Geometry check sheet. Reference: the model listing, model coordinates, mm. Coordinates: 2 decimals unless noted, no trailing zeros. Order: outer loops, then holes, each group sorted by start corner. A loop starts at its lowest first (then second) coordinate and runs counter-clockwise, first axis right, second up. Notation, with made-up numbers: M 42.25,53 L 91.25,53 A18 ccw 91.25,83 Z; hole C -27,-10 d9. An arc over 180 degrees is marked long. One line per item, written item: value. Start each with the question number.
1) Sectioned sample at A-A, the plane x = 0. Enter the section's corners in (y, z) (3 decimals), then the cut area to 3 significant figures.
2) Sectioned sample at B-B, the plane z = 0. Enter the section's corners in (x, y) (3 decimals), then the cut area to 3 significant figures.
3) Go/stop test with flat-tipped pins: P1, Ø2, axis at y = 1, z = -3.5, coming from the -X side; P2, Ø1, axis at y = -1, z = -2.5, coming from the +X side; P3, Ø1, axis at x = 1, y = 0.5, coming from the +Z side. Record where each tip stops, or that it passes through.
4) Thickness scan on L1, parallel to Z at x = 0, y = -0.2; L2, parallel to X at y = -1.1, z = 1.5. Record the ranges inside material, lowest first. Write a range as from..to.
5) Sectioned sample at C-C, the plane y = -0.15. Enter the section's corners in (x, z).
6) Draft check along X on faces 1 (the cylindrical face through (0, 0, 2)), 2 (the cylindrical face through (-1.08, 0.02, 4.88)), 3 (the flat face through (2, -2, 2)). Enter one of: pulls with the +X half, pulls with the -X half, needs draft (parallel to the pull), parting line crosses it, or undercut.
```python
from build123d import *

# Parameters (mm, degrees)
SKETCH1_R               = 5
BOSS_EXTRUDE1_DEPTH     = 2
SKETCH2_R               = 2
CUT_EXTRUDE1_DEPTH      = 3
CUT_EXTRUDE1_DEPTH_BACK = 3
FILLET1_R               = 0.375


with BuildPart() as part:
    # Sketch1 → Boss-Extrude1 (new body, symmetric)
    with BuildSketch(Plane(origin=(0, 0, 0), x_dir=(1, 0, 0), z_dir=(0, 1, 0))):
        Circle(SKETCH1_R)
    extrude(amount=BOSS_EXTRUDE1_DEPTH, both=True)

    # Sketch2 → Cut-Extrude1 (cut, two sides)
    with BuildSketch(Plane(origin=(0, 0, 0), x_dir=(1, 0, 0), z_dir=(0, 1, 0))) as cut_extrude1_sk:
        Circle(SKETCH2_R)
    extrude(amount=CUT_EXTRUDE1_DEPTH, mode=Mode.SUBTRACT)
    extrude(cut_extrude1_sk.sketch, amount=-CUT_EXTRUDE1_DEPTH_BACK, mode=Mode.SUBTRACT)

    # Fillet1
    fillet1_edges = [part.edges().sort_by_distance(p)[0] for p in [
        (-5, -2, 0),
        (-5, 2, 0),
        (-2, -2, 0),
        (-2, 2, 0),
    ]]
    fillet(fillet1_edges, radius=FILLET1_R)


solid = part.part
```
Final values:
1. outline: M -2,-4.625 A0.375 ccw -1.625,-5 L 1.625,-5 A0.375 ccw 2,-4.625 L 2,-2.375 A0.375 ccw 1.625,-2 L -1.625,-2 A0.375 ccw -2,-2.375 Z; M -2,2.375 A0.375 ccw -1.625,2 L 1.625,2 A0.375 ccw 2,2.375 L 2,4.625 A0.375 ccw 1.625,5 L -1.625,5 A0.375 ccw -2,4.625 Z
1. area: 23.8 mm^2
2. outline: M -5,-1.625 A0.375 ccw -4.625,-2 L -2.375,-2 A0.375 ccw -2,-1.625 L -2,1.625 A0.375 ccw -2.375,2 L -4.625,2 A0.375 ccw -5,1.625 Z; M 2,-1.625 A0.375 ccw 2.375,-2 L 4.625,-2 A0.375 ccw 5,-1.625 L 5,1.625 A0.375 ccw 4.625,2 L 2.375,2 A0.375 ccw 2,1.625 Z
2. area: 23.8 mm^2
3. P1: stops at x = -4.33
3. P2: stops at x = 4.58
3. P3: stops at z = 4.97
4. L1: z = -5..-2, 2..5
4. L2: x = -4.77..-1.32, 1.32..4.77
5. outline: C 0,0 d10; hole C 0,0 d4
6. face 1: undercut
6. face 2: parting line crosses it
6. face 3: needs draft
